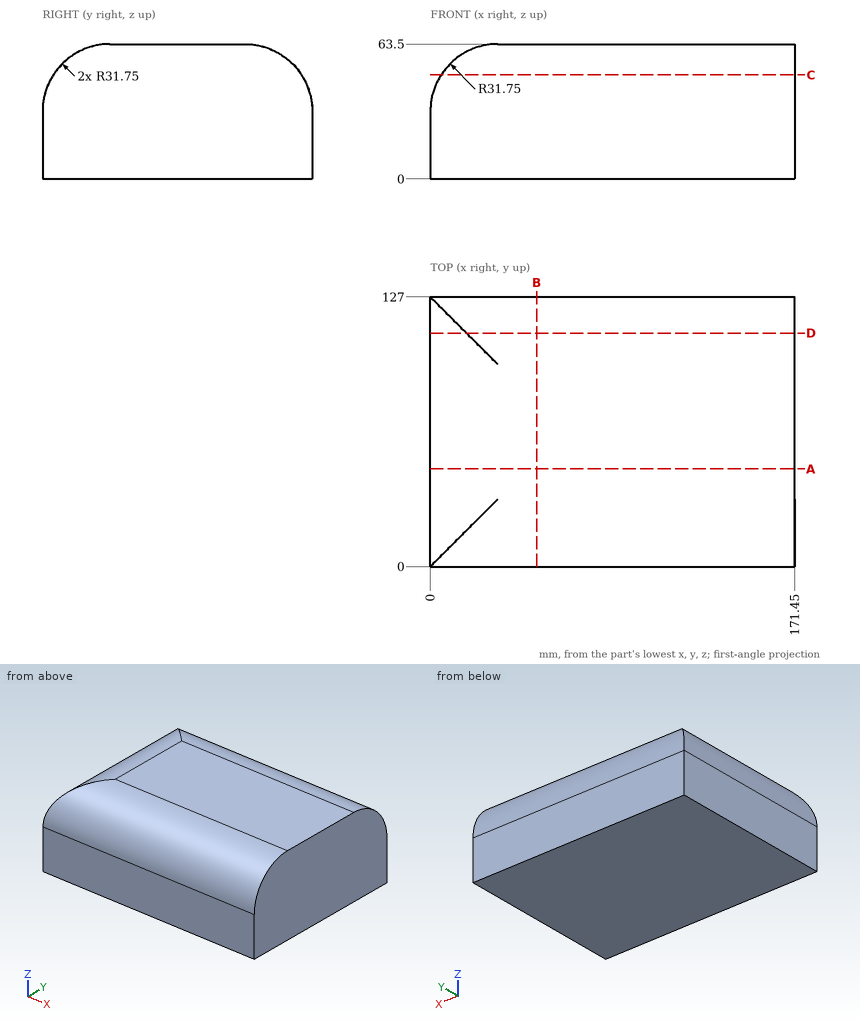
The figure shows three views and two pictorial views of one solid part (mm, origin at its lowest corner). Answer the questions. Give positions to 0.01 mm unless a question says otherwise; leave off trailing zeros. Loops run counter-clockwise (first coordinate to the right, second up) from the corner with the lowest first, then second, coordinate; pieces in that order, holes last. Notation, with made-up numbers: (-3.75, 60.25) -> (47.25, 60.25) arc R22 cw to (47.25, 81.25) -> close; hole circle Ø6 at (62.25, 57.25). An arc over 180 degrees is marked (long way). Use a Markdown table: item, result. Add a question column.
1. Section C-C on z = 49 is taken. Determine the outline of the cut face in (x, y).
2. Flat-ended cylindrical pins translate along their axes: pin 1 Ø6 at (x, z) = (49.5, 33) entering from +Y; pin 2 Ø3 at (x, z) = (107, 39) entering from +Y (3 decimals); pin 3 Ø2 at (y, z) = (83, 52) entering from -X; pin 4 Ø4 at (y, z) = (40.5, 40) entering from -X. Find the tip coordinate at first contact, or state that the pin passes through.
3. Find the intervals of material crossed by probe 1 along X at (y, z) = (61.5, 53); probe 2 along Z at (x, y) = (73.5, 19); probe 3 along Y at (x, z) = (58, 45), in increasing order.
4. Section A-A on y = 46 is taken. Determine the outline of the cut face in (x, z), and give its area (3 significant figures).
5. Section D-D on y = 110 is taken. Determine the outline of the cut face in (x, z), and give its area (3 significant figures).
6. Section B-B on x = 50 is taken. Determine the outline of the cut face in (y, z).
Results below:
| question | item | result |
|---|---|---|
| 1 | outline | (5.09, 5.09) -> (171.45, 5.09) -> (171.45, 121.91) -> (5.09, 121.91) -> close |
| 2 | pin 1 | stops at y = 127 |
| 2 | pin 2 | stops at y = 126.475 |
| 2 | pin 3 | stops at x = 6.5 |
| 2 | pin 4 | stops at x = 0.62 |
| 3 | probe 1 | x = 8.16 to 171.45 |
| 3 | probe 2 | z = 0 to 60.83 |
| 3 | probe 3 | y = 2.9 to 124.1 |
| 4 | outline | (0, 0) -> (171.45, 0) -> (171.45, 63.5) -> (31.75, 63.5) arc R31.75 ccw to (0, 31.75) -> close |
| 4 | area | 10,700 mm^2 |
| 5 | outline | (0, 0) -> (171.45, 0) -> (171.45, 59.87) -> (17, 59.87) arc R31.75 ccw to (0, 31.75) -> close |
| 5 | area | 10,100 mm^2 |
| 6 | outline | (0, 0) -> (127, 0) -> (127, 31.75) arc R31.75 ccw to (95.25, 63.5) -> (31.75, 63.5) arc R31.75 ccw to (0, 31.75) -> close |
